Could you check a few things on this model? Use its own coordinates, in mm. Face numbers are marked on the shaded views. A direction names the side the tool comes from. Coordinates: 2 decimals unless noted, no trailing zeros. Order: outer loops, then holes, each group sorted by start corner. A loop starts at its lowest first (then second) coordinate and runs counter-clockwise, first axis right, second up. Notation, with made-up numbers: M 20,21.5 L 66,21.5 A28 cw 66,49.5 Z; hole C 56,-27 d9. An arc over 180 degrees is marked long. One line per question, with ' | ' between items. Start each with the question number.
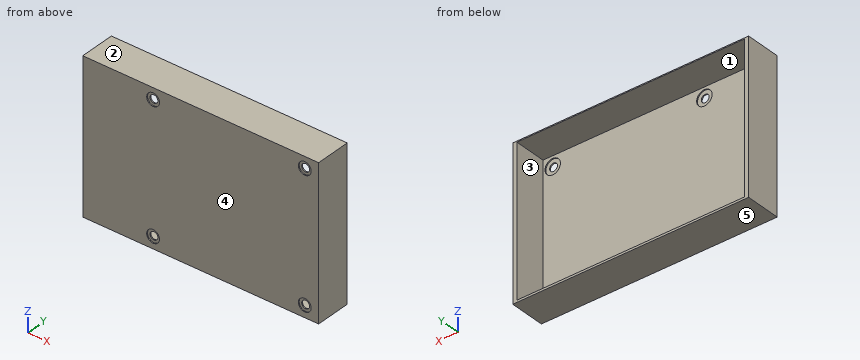
from build123d import *

# Parameters (mm, degrees)
SKIZZE1_W                       = 90.2
SKIZZE1_H                       = 57.8
SKIZZE1_W_2                     = 87
SKIZZE1_H_2                     = 56.6
AUFSATZ_LINEAR_AUSTRAGEN1_DEPTH = 12.3
SKIZZE2_W                       = 90.2
SKIZZE2_H                       = 57.8
AUFSATZ_LINEAR_AUSTRAGEN2_DEPTH = 1.2
SKIZZE3_R                       = 1.5
SCHNITT_LINEAR_AUSTRAGEN1_DEPTH = 1.2
SKIZZE4_R                       = 2.45
SCHNITT_LINEAR_AUSTRAGEN2_DEPTH = 0.4
SKIZZE5_R                       = 2.95
SCHNITT_LINEAR_AUSTRAGEN3_DEPTH = 0.4


with BuildPart() as part:
    # Skizze1 → Aufsatz-Linear austragen1 (new body)
    with BuildSketch(Plane(origin=(0, 0, 0), x_dir=(1, 0, 0), z_dir=(0, 1, 0))):
        with Locations((45.1, 28.9)):
            Rectangle(SKIZZE1_W, SKIZZE1_H)
        with Locations((45.1, 28.7)):
            Rectangle(SKIZZE1_W_2, SKIZZE1_H_2, mode=Mode.SUBTRACT)
    extrude(amount=AUFSATZ_LINEAR_AUSTRAGEN1_DEPTH)

    # Skizze2 → Aufsatz-Linear austragen2 (add)
    with BuildSketch(Plane(origin=(0, 0, 0), x_dir=(1, 0, 0), z_dir=(0, 1, 0))):
        with Locations((45.1, 28.9)):
            Rectangle(SKIZZE2_W, SKIZZE2_H)
    extrude(amount=-AUFSATZ_LINEAR_AUSTRAGEN2_DEPTH)

    # Skizze3 → Schnitt-Linear austragen1 (cut)
    with BuildSketch(Plane(origin=(0, 0, 0), x_dir=(1, 0, 0), z_dir=(0, 1, 0))):
        with Locations(Location((84.9, 53.3, 0), (0, 0, 270))):
            Circle(SKIZZE3_R)
        with Locations(Location((26.9, 53.3, 0), (0, 0, 270))):
            Circle(SKIZZE3_R)
        with Locations(Location((84.9, 4.3, 0), (0, 0, 270))):
            Circle(SKIZZE3_R)
        with Locations(Location((26.9, 4.3, 0), (0, 0, 270))):
            Circle(SKIZZE3_R)
    extrude(amount=-SCHNITT_LINEAR_AUSTRAGEN1_DEPTH, mode=Mode.SUBTRACT)

    # Skizze4 → Schnitt-Linear austragen2 (cut)
    with BuildSketch(Plane(origin=(0, -1.2, 0), x_dir=(1, 0, 0), z_dir=(0, 1, 0))):
        with Locations(Location((84.9, 53.3, 0), (0, 0, 270))):
            Circle(SKIZZE4_R)
        with Locations(Location((26.9, 53.3, 0), (0, 0, 270))):
            Circle(SKIZZE4_R)
        with Locations(Location((84.9, 4.3, 0), (0, 0, 270))):
            Circle(SKIZZE4_R)
        with Locations(Location((26.9, 4.3, 0), (0, 0, 270))):
            Circle(SKIZZE4_R)
    extrude(amount=SCHNITT_LINEAR_AUSTRAGEN2_DEPTH, mode=Mode.SUBTRACT)

    # Skizze5 → Schnitt-Linear austragen3 (cut)
    with BuildSketch(Plane(origin=(0, 0, 0), x_dir=(1, 0, 0), z_dir=(0, 1, 0))):
        with Locations(Location((84.9, 53.3, 0), (0, 0, 270))):
            Circle(SKIZZE5_R)
        with Locations(Location((26.9, 53.3, 0), (0, 0, 270))):
            Circle(SKIZZE5_R)
        with Locations(Location((84.9, 4.3, 0), (0, 0, 270))):
            Circle(SKIZZE5_R)
        with Locations(Location((26.9, 4.3, 0), (0, 0, 270))):
            Circle(SKIZZE5_R)
    extrude(amount=-SCHNITT_LINEAR_AUSTRAGEN3_DEPTH, mode=Mode.SUBTRACT)


solid = part.part
(1) If I drill on line 1 along Z through (x, y) = (84.9, -0.55); line 2 along X through (y, z) = (-1, -53.3); line 3 along X through (y, z) = (-0.3, -4.3), over which ranges is the centre line in solid material (lowest first)? Write a range as from..to.
(2) Imagine slicing it at A-A, the plane x = 84.9. Count the separate pieces of the cut face and the enclosed holes in it, plus the area to 3 significant figures.
(3) Imagine slicing it at C-C, the plane y = 8.5. Write out the boundary of the cut face in (x, z).
(4) For P1, Ø4, axis at x = 26.9, z = -53.3, coming from the +Y side; P2, Ø6, axis at x = 9, z = -31.5, coming from the +Y side, each with a flat end and sliding along its axis, tell me the tip position at first contact or that it passes through.
(5) On a 3-axis mill with a long thin cutter (end or side, diameter ignored), from which of +Z, -Z, +X, -X, +Y, -Y can I reach the whole of each face in a straight line? I mean the marked faces 1 and 2. Say none if no direction works.
(6) We'd pull the mould along Z, two halves only. Please class the marked faces 3, 4 and 5: +Z half, -Z half, draft (parallel to the pull), parting line (faces both ways), or undercut.
(7) Imagine slicing it at D-D, the plane x = 37. Write out the boundary of the cut face in (y, z).
Answers:
1) line 1: -57.8..-54.8, -51.8..-5.8, -2.8..0 | line 2: 0..24.45, 29.35..82.45, 87.35..90.2 | line 3: 0..23.95, 29.85..81.95, 87.85..90.2
2) separate pieces: 3 | enclosed holes: 0 | area: 73.1 mm²
3) outline: M 0,-57.8 L 90.2,-57.8 L 90.2,0 L 0,0 Z; hole M 1.6,-57 L 88.6,-57 L 88.6,-0.4 L 1.6,-0.4 Z
4) P1: y = -0.4 | P2: y = 0
5) face 1: +Y | face 2: +Z, +X, -X, +Y, -Y
6) face 3: undercut | face 4: draft | face 5: -Z half
7) outline: M -1.2,-57.8 L 12.3,-57.8 L 12.3,-57 L 0,-57 L 0,-0.4 L 12.3,-0.4 L 12.3,0 L -1.2,0 Z
